Check sheet for the modelled part. Datum: model origin and axes. Units: mm. Give positions to 0.01 mm unless a question says otherwise; leave off trailing zeros. Order: outer loops, then holes, each group sorted by start corner. A loop starts at its lowest first (then second) coordinate and runs counter-clockwise, first axis right, second up. Notation, with made-up numbers: (87.5, -29) -> (103.5, -29) arc R11 ccw to (103.5, -25) -> close; hole circle Ø5 at (-29.5, 9). An arc over 180 degrees is marked (long way). Write each question's results on one line, items separated by ' | '.
from build123d import *

# Parameters (mm, degrees)
EXTRUDE_1_DEPTH     = 440
SKETCH_2_R          = 1.75
CUT_EXTRUDE_3_DEPTH = 440
SKETCH_3_R          = 3.25
CUT_EXTRUDE_4_DEPTH = 3.5


with BuildPart() as part:
    # 草图1 → 凸台-拉伸1 (new body)
    with BuildSketch(Plane.XY):
        Polygon((0, 0), (-9, 0), (-9, 4.208125846), (-8.343397225, 4.785997189), (-8.055092033, 4.785997189), (-8.055092033, 5.184529149), (-8.343397225, 5.184529149), (-9, 5.762400492), (-9, 6.5), (0, 6.5), (0, 5.762400492), (-0.656602775, 5.184529149), (-0.944907967, 5.184529149), (-0.944907967, 4.785997189), (-0.656602775, 4.785997189), (0, 4.208125846), align=None)
    extrude(amount=EXTRUDE_1_DEPTH)

    # 草图2 → 切除-拉伸3 (cut)
    with BuildSketch(Plane(origin=(0, 6.5, 0), x_dir=(1, 0, 0), z_dir=(0, 1, 0))):
        with Locations(Location((-4.5, -6.942433545, 0), (0, 0, 180))):
            Circle(SKETCH_2_R)
        with Locations(Location((-4.5, -26.942433545, 0), (0, 0, 180))):
            Circle(SKETCH_2_R)
        with Locations(Location((-4.5, -46.942433545, 0), (0, 0, 180))):
            Circle(SKETCH_2_R)
        with Locations(Location((-4.5, -66.942433545, 0), (0, 0, 180))):
            Circle(SKETCH_2_R)
        with Locations(Location((-4.5, -86.942433545, 0), (0, 0, 180))):
            Circle(SKETCH_2_R)
        with Locations(Location((-4.5, -106.942433545, 0), (0, 0, 180))):
            Circle(SKETCH_2_R)
        with Locations(Location((-4.5, -126.942433545, 0), (0, 0, 180))):
            Circle(SKETCH_2_R)
        with Locations(Location((-4.5, -146.942433545, 0), (0, 0, 180))):
            Circle(SKETCH_2_R)
        with Locations(Location((-4.5, -166.942433545, 0), (0, 0, 180))):
            Circle(SKETCH_2_R)
        with Locations(Location((-4.5, -186.942433545, 0), (0, 0, 180))):
            Circle(SKETCH_2_R)
        with Locations(Location((-4.5, -206.942433545, 0), (0, 0, 180))):
            Circle(SKETCH_2_R)
        with Locations(Location((-4.5, -226.942433545, 0), (0, 0, 180))):
            Circle(SKETCH_2_R)
        with Locations(Location((-4.5, -246.942433545, 0), (0, 0, 180))):
            Circle(SKETCH_2_R)
        with Locations(Location((-4.5, -266.942433545, 0), (0, 0, 180))):
            Circle(SKETCH_2_R)
        with Locations(Location((-4.5, -286.942433545, 0), (0, 0, 180))):
            Circle(SKETCH_2_R)
        with Locations(Location((-4.5, -306.942433545, 0), (0, 0, 180))):
            Circle(SKETCH_2_R)
        with Locations(Location((-4.5, -326.942433545, 0), (0, 0, 180))):
            Circle(SKETCH_2_R)
        with Locations(Location((-4.5, -346.942433545, 0), (0, 0, 180))):
            Circle(SKETCH_2_R)
        with Locations(Location((-4.5, -366.942433545, 0), (0, 0, 180))):
            Circle(SKETCH_2_R)
        with Locations(Location((-4.5, -386.942433545, 0), (0, 0, 180))):
            Circle(SKETCH_2_R)
        with Locations(Location((-4.5, -406.942433545, 0), (0, 0, 180))):
            Circle(SKETCH_2_R)
        with Locations(Location((-4.5, -426.942433545, 0), (0, 0, 180))):
            Circle(SKETCH_2_R)
    extrude(amount=-CUT_EXTRUDE_3_DEPTH, mode=Mode.SUBTRACT)

    # 草图3 → 切除-拉伸4 (cut)
    with BuildSketch(Plane(origin=(0, 6.5, 0), x_dir=(1, 0, 0), z_dir=(0, 1, 0))):
        with Locations(Location((-4.5, -6.942433545, 0), (0, 0, 180))):
            Circle(SKETCH_3_R)
        with Locations(Location((-4.5, -26.942433545, 0), (0, 0, 180))):
            Circle(SKETCH_3_R)
        with Locations(Location((-4.5, -46.942433545, 0), (0, 0, 180))):
            Circle(SKETCH_3_R)
        with Locations(Location((-4.5, -66.942433545, 0), (0, 0, 180))):
            Circle(SKETCH_3_R)
        with Locations(Location((-4.5, -86.942433545, 0), (0, 0, 180))):
            Circle(SKETCH_3_R)
        with Locations(Location((-4.5, -106.942433545, 0), (0, 0, 180))):
            Circle(SKETCH_3_R)
        with Locations(Location((-4.5, -126.942433545, 0), (0, 0, 180))):
            Circle(SKETCH_3_R)
        with Locations(Location((-4.5, -146.942433545, 0), (0, 0, 180))):
            Circle(SKETCH_3_R)
        with Locations(Location((-4.5, -166.942433545, 0), (0, 0, 180))):
            Circle(SKETCH_3_R)
        with Locations(Location((-4.5, -186.942433545, 0), (0, 0, 180))):
            Circle(SKETCH_3_R)
        with Locations(Location((-4.5, -206.942433545, 0), (0, 0, 180))):
            Circle(SKETCH_3_R)
        with Locations(Location((-4.5, -226.942433545, 0), (0, 0, 180))):
            Circle(SKETCH_3_R)
        with Locations(Location((-4.5, -246.942433545, 0), (0, 0, 180))):
            Circle(SKETCH_3_R)
        with Locations(Location((-4.5, -266.942433545, 0), (0, 0, 180))):
            Circle(SKETCH_3_R)
        with Locations(Location((-4.5, -286.942433545, 0), (0, 0, 180))):
            Circle(SKETCH_3_R)
        with Locations(Location((-4.5, -306.942433545, 0), (0, 0, 180))):
            Circle(SKETCH_3_R)
        with Locations(Location((-4.5, -326.942433545, 0), (0, 0, 180))):
            Circle(SKETCH_3_R)
        with Locations(Location((-4.5, -346.942433545, 0), (0, 0, 180))):
            Circle(SKETCH_3_R)
        with Locations(Location((-4.5, -366.942433545, 0), (0, 0, 180))):
            Circle(SKETCH_3_R)
        with Locations(Location((-4.5, -386.942433545, 0), (0, 0, 180))):
            Circle(SKETCH_3_R)
        with Locations(Location((-4.5, -406.942433545, 0), (0, 0, 180))):
            Circle(SKETCH_3_R)
        with Locations(Location((-4.5, -426.942433545, 0), (0, 0, 180))):
            Circle(SKETCH_3_R)
        with Locations((-4.5, -446.942433545)):
            Circle(SKETCH_3_R)
        with Locations((-4.5, -466.942433545)):
            Circle(SKETCH_3_R)
        with Locations((-4.5, -486.942433545)):
            Circle(SKETCH_3_R)
        with Locations((-4.5, -506.942433545)):
            Circle(SKETCH_3_R)
        with Locations((-4.5, -526.942433545)):
            Circle(SKETCH_3_R)
        with Locations((-4.5, -546.942433545)):
            Circle(SKETCH_3_R)
        with Locations((-4.5, -566.942433545)):
            Circle(SKETCH_3_R)
        with Locations((-4.5, -586.942433545)):
            Circle(SKETCH_3_R)
        with Locations((-4.5, -606.942433545)):
            Circle(SKETCH_3_R)
    extrude(amount=-CUT_EXTRUDE_4_DEPTH, mode=Mode.SUBTRACT)


solid = part.part
1. Section check A-A on x = -4.5. Give the number of separate pieces and of enclosed holes in the cut face, then the cut area to 3 significant figures.
Verdict:
separate pieces: 23 | enclosed holes: 0 | area: 2,130 mm^2
2. Material ranges on probe 1 along X at (y, z) = (3.75, 226.5); probe 2 along Y at (x, z) = (-0.75, 412); probe 3 along Y at (x, z) = (-4, 209.5), recorded low to high. Write a range as from..to.
Verdict:
probe 1: x = -9..-7.72, -1.28..0 | probe 2: y = 0..4.79, 5.18..6.5 | probe 3: y = 0..3
3. Gauge pin test, flat ends, axial feed: pin 1 Ø2 at (x, z) = (-6, 386.5) entering from +Y; pin 2 Ø2 at (x, z) = (-4.5, 426.94) entering from -Y. Record the tip position at first contact, or that the pin passes through.
Verdict:
pin 1: stops at y = 3 | pin 2: passes through
4. Section check B-B on z = 180. Record the cut outline in (x, y).
Verdict:
outline: (-9, 0) -> (0, 0) -> (0, 4.21) -> (-0.66, 4.79) -> (-0.94, 4.79) -> (-0.94, 5.18) -> (-0.66, 5.18) -> (0, 5.76) -> (0, 6.5) -> (-9, 6.5) -> (-9, 5.76) -> (-8.34, 5.18) -> (-8.06, 5.18) -> (-8.06, 4.79) -> (-8.34, 4.79) -> (-9, 4.21) -> close
